Answer from the drawing. Dimensions are ordinates in mm from the lowest x, y and z of the part. Coordinates: 2 decimals unless noted, no trailing zeros. Write each loop counter-clockwise with the first axis right and the second up, starting at its lowest first coordinate (ties: lowest second). Pieces come first, ordered by that corner, then holes.
(1) For a pull along Z with two mould halves and no side action, classify the marked faces 1, 2, 3 and 4 as +Z half, -Z half, draft (parallel to the pull), parting line (faces both ways), or undercut.
(2) Straight lines are drawn through the part: line 1 (Z direction, x = 6.6, y = 2); line 2 (Z direction, x = 13.9, y = 5); line 3 (X direction, y = 3.25, z = 13.5). For each, find the intervals that lie inside material, in ascending order.
(3) The part is cut by section A-A on x = 6.6. Determine the outline of the cut face in (y, z), plus the area to 3 significant figures.
(4) The part is cut by section C-C on y = 4.5. Determine the outline of the cut face in (x, z).
(5) Given P1, Ø1.8, axis at x = 13.9, z = 14.5, coming from the -Y side, flat-ended and moving along its own axis, determine where the tip first touches the part or whether it passes through.
(6) The part is cut by section B-B on z = 2. Determine the outline of the cut face in (x, y).
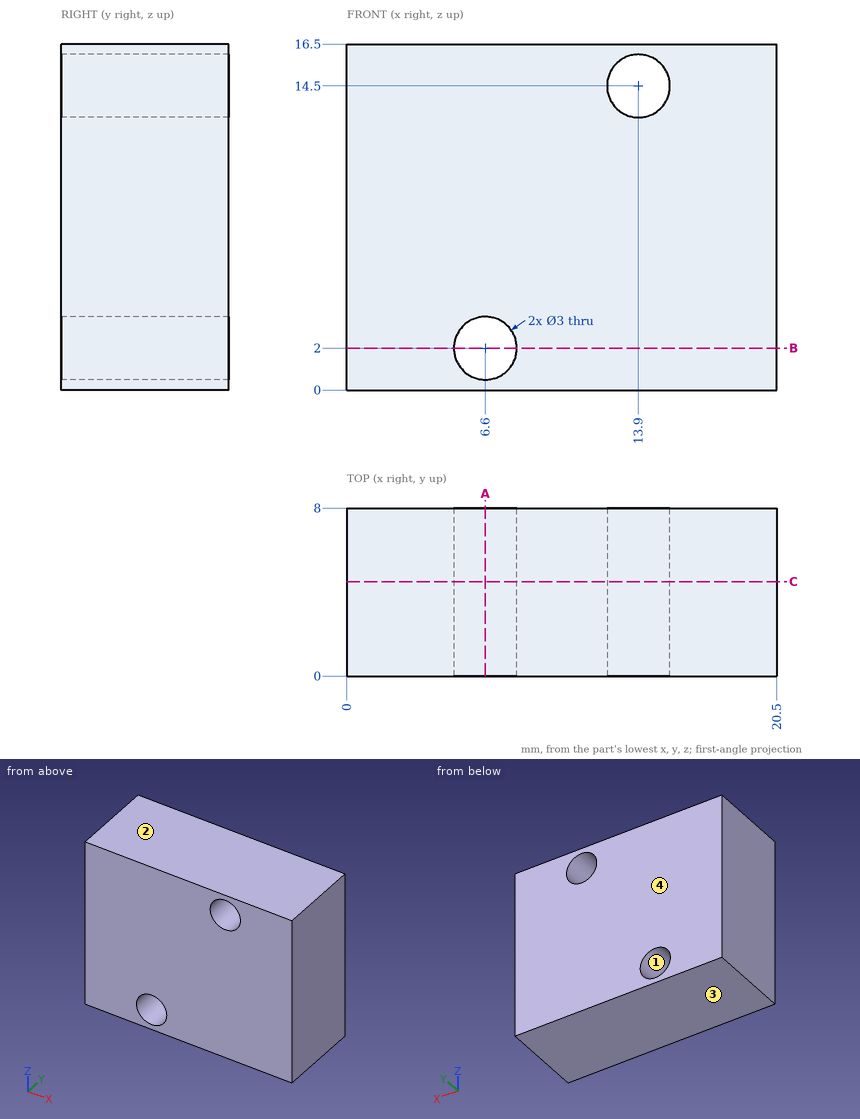
Model answer:
1. face 1: undercut
1. face 2: +Z half
1. face 3: -Z half
1. face 4: draft
2. line 1: z = 0 to 0.5, 3.5 to 16.5
2. line 2: z = 0 to 13, 16 to 16.5
2. line 3: x = 0 to 12.78, 15.02 to 20.5
3. outline: (0, 0) - (8, 0) - (8, 0.5) - (0, 0.5) - close; (0, 3.5) - (8, 3.5) - (8, 16.5) - (0, 16.5) - close
3. area: 108 mm2
4. outline: (0, 0) - (20.5, 0) - (20.5, 16.5) - (0, 16.5) - close; hole circle Ø3 at (6.6, 2); hole circle Ø3 at (13.9, 14.5)
5. P1: passes through
6. outline: (0, 0) - (5.1, 0) - (5.1, 8) - (0, 8) - close; (8.1, 0) - (20.5, 0) - (20.5, 8) - (8.1, 8) - close
